The model under review builds one solid part; all positions refer to its coordinate system, in mm. A direction names the side the tool comes from. Round coordinates to 2 decimals unless told otherwise and drop trailing zeros. Write each loop counter-clockwise with the first axis right and the second up, starting at its lowest first coordinate (ties: lowest second). Pieces come first, ordered by that corner, then holes. Notation, with made-up numbers: M -10,-7 L -2,-7 A26 ccw -2,22 Z; hole C 18.25,8.5 d4. An arc over 180 degrees is marked long. Write item = value, one per line. Start each with the question number.
Item 1: Take a section at C-C, the plane y = -8.5. Give the boundary of the cut face in (x, z), plus the area to 3 significant figures.
Item 2: Take a section at A-A, the plane y = 0. Give the boundary of the cut face in (x, z), plus the area to 3 significant figures.
Item 3: Take a section at B-B, the plane x = 0. Give the boundary of the cut face in (y, z).
Item 4: For pin 1 Ø2 at (y, z) = (-3.5, 3) entering from -X; pin 2 Ø2.5 at (y, z) = (14, 3.5) entering from -X, all flat-tipped, find the tip position at first contact; note any pin that passes through.
Item 5: Take a section at D-D, the plane z = 3. Give the number of separate pieces and of enclosed holes in the cut face, plus the area to 3 significant figures.
Item 6: The part is to be moulded in two halves that separate along Y. For faces 3 (the flat face through (29.108, 11, 3)), 4 (the flat face through (-1, -5, 0)), say which applies: +Y half, -Y half, draft (parallel to the pull), parting line (faces both ways), or undercut.
Item 7: Tool access review of faces 1 (the flat face through (82.77, 11.16, 2.54)), 2 (the flat face through (-103.428, 21, 2)): name each direction out of +Z, -Z, +X, -X, +Y, -Y from which nothing blocks a thin tool from reaching the whole face with its end or side.
Item 8: To check wall thickness, follow line 1 along Y through (x, z) = (-8, 2.15); line 2 along Y through (x, z) = (32, 1.65); line 3 along X through (y, z) = (1, 1.3). State the ranges of each line that lie inside material, in increasing order.
from build123d import *

# Parameters (mm, degrees)
SKETCH1_W           = 206.856
SKETCH1_H           = 48
SKETCH1_R           = 2.5
BOSS_EXTRUDE1_DEPTH = 5
SKETCH2_R           = 17.5
SKETCH2_W           = 25
SKETCH2_H           = 12.5
CUT_EXTRUDE1_DEPTH  = 107.293702466


with BuildPart() as part:
    # Sketch1 → Boss-Extrude1 (new body)
    with BuildSketch(Plane.XY):
        Rectangle(SKETCH1_W, SKETCH1_H)
        Circle(SKETCH1_R, mode=Mode.SUBTRACT)
        with Locations((32, 0)):
            Circle(SKETCH1_R, mode=Mode.SUBTRACT)
        with Locations((-32, 0)):
            Circle(SKETCH1_R, mode=Mode.SUBTRACT)
    extrude(amount=BOSS_EXTRUDE1_DEPTH)

    # Sketch2 → Cut-Extrude1 (cut, through all)
    with BuildSketch(Plane.XY.offset(5)):
        with Locations((103.428, 0)):
            Circle(SKETCH2_R)
        Polygon((89.108194847, 17.5), (36.608194847, 17.5), (36.608194847, 5), (76.608194847, 5), align=None)
        with Locations((16.608194847, 11.25)):
            Rectangle(SKETCH2_W, SKETCH2_H)
        Polygon((89.108194847, -17.5), (36.608194847, -17.5), (36.608194847, -5), (76.608194847, -5), align=None)
        with Locations((16.608194847, -11.25)):
            Rectangle(SKETCH2_W, SKETCH2_H)
    cut_extrude1 = extrude(amount=-CUT_EXTRUDE1_DEPTH, mode=Mode.SUBTRACT)

    # Mirror1: Cut-Extrude1 across plane
    add(cut_extrude1.mirror(Plane(origin=(0, 0, 0), x_dir=(0, 0, 1), z_dir=(1, 0, 0))), mode=Mode.SUBTRACT)


solid = part.part
Response values:
q1.outline = M -88.13,0 L -80.11,0 L -80.11,5 L -88.13,5 Z; M -36.61,0 L -29.11,0 L -29.11,5 L -36.61,5 Z; M -4.11,0 L 4.11,0 L 4.11,5 L -4.11,5 Z; M 29.11,0 L 36.61,0 L 36.61,5 L 29.11,5 Z; M 80.11,0 L 88.13,0 L 88.13,5 L 80.11,5 Z
q1.area = 196 mm2
q2.outline = M -85.93,0 L -34.5,0 L -34.5,5 L -85.93,5 Z; M -29.5,0 L -2.5,0 L -2.5,5 L -29.5,5 Z; M 2.5,0 L 29.5,0 L 29.5,5 L 2.5,5 Z; M 34.5,0 L 85.93,0 L 85.93,5 L 34.5,5 Z
q2.area = 784 mm2
q3.outline = M -24,0 L -2.5,0 L -2.5,5 L -24,5 Z; M 2.5,0 L 24,0 L 24,5 L 2.5,5 Z
q4.pin_1 = -86.52
q4.pin_2 = -94.84
q5.separate_pieces = 1
q5.enclosed_holes = 11
q5.area = 5,350 mm2
q6.face_3 = undercut
q6.face_4 = draft
q7.face_1 = +Z, -Z
q7.face_2 = +Z, -Z, -X, +Y, -Y
q8.line_1 = -24 to -17.5, -5 to 5, 17.5 to 24
q8.line_2 = -24 to -2.5, 2.5 to 24
q8.line_3 = -85.96 to -34.29, -29.71 to -2.29, 2.29 to 29.71, 34.29 to 85.96
